The model under review builds one solid part; all positions refer to its coordinate system, in mm. A direction names the side the tool comes from. Round coordinates to 2 decimals unless told otherwise and drop trailing zeros. Write each loop counter-clockwise with the first axis right and the second up, starting at its lowest first coordinate (ties: lowest second). Pieces come first, ordered by that corner, then holes. Notation, with made-up numbers: (27, -39.75) - (35, -39.75) arc R13 ccw to (35, -32.75) - close; hole circle Ø1 at (84, 23.5). An arc over 180 degrees is marked (long way). Use one line per item in the form item = value.
from build123d import *

# Parameters (mm, degrees)
BOSS_EXTRUDE1_DEPTH  = 3
SKETCH1_3_R          = 1.6
CUT_EXTRUDE1_DEPTH   = 219.249429386
MNTPATT_LNDGEAR_D    = 3.4
MNTPATT_REARARM_D    = 3.4
MNTPATT_FOREARM_D    = 3.4
FILLET1_R            = 5
FILLET2_R            = 2
M3_CLEARANCE_HOLE4_D = 3.4


with BuildPart() as part:
    # Sketch1 → Boss-Extrude1 (new body)
    with BuildSketch(Plane.XY):
        Polygon((0, 0), (19, 0), (21.979383981, 2.5), (40.979383981, 2.5), (62.987827091, -27.242703843), (50.343119944, -50.531357328), (50.343119944, -94.031357328), (90.343119944, -163.313389631), (66.562485529, -184.725569035), (51.780413009, -178.602634117), (41.565626765, -198.650280911), (29.565626765, -198.650280911), (29.565626765, -177.650280911), (0, -177.650280911), align=None)
    boss_extrude1 = extrude(amount=BOSS_EXTRUDE1_DEPTH)

    # Sketch1<3> → Cut-Extrude1 (cut, through all)
    with BuildSketch(Plane.XY):
        with Locations((6, -4)):
            Circle(SKETCH1_3_R)
        with Locations((48.043119944, -104.047640471)):
            Circle(SKETCH1_3_R)
        with Locations((53.591147617, -139.888439508)):
            Circle(SKETCH1_3_R)
        with Locations((36.065626765, -194.650280911)):
            Circle(SKETCH1_3_R)
        with Locations((24, -172.650280911)):
            Circle(SKETCH1_3_R)
        with Locations((9, -170.650280911)):
            Circle(SKETCH1_3_R)
        with Locations((15.778522962, -34.052256336)):
            Circle(SKETCH1_3_R)
    cut_extrude1 = extrude(amount=CUT_EXTRUDE1_DEPTH, mode=Mode.SUBTRACT)

    # MntPatt-Lndgear (through all)
    with Locations(Plane.XY.offset(3)):
        with Locations((33.343119944, -56.83261542), (41.343119944, -56.83261542), (33.343119944, -87.83261542), (41.343119944, -87.83261542)):
            mntpatt_lndgear = Hole(MNTPATT_LNDGEAR_D / 2)

    # MntPatt-RearArm (through all)
    with Locations(Plane.XY.offset(3)):
        with Locations((55.826108536, -26.810648111), (50.472703455, -19.575936365)):
            mntpatt_reararm = Hole(MNTPATT_REARARM_D / 2)

    # MntPatt_ForeArm (through all)
    with Locations(Plane.XY.offset(3)):
        with Locations((71.326111319, -173.035401095), (64.63780789, -179.057576552)):
            mntpatt_forearm = Hole(MNTPATT_FOREARM_D / 2)

    # Mirror2: Boss-Extrude1, Cut-Extrude1, MntPatt-Lndgear, MntPatt-RearArm, MntPatt_ForeArm across plane
    add(boss_extrude1.mirror(Plane(origin=(0, 0, 3), x_dir=(0, 0, 1), z_dir=(1, 0, 0))))
    add(cut_extrude1.mirror(Plane(origin=(0, 0, 3), x_dir=(0, 0, 1), z_dir=(1, 0, 0))), mode=Mode.SUBTRACT)
    add(mntpatt_lndgear.mirror(Plane(origin=(0, 0, 3), x_dir=(0, 0, 1), z_dir=(1, 0, 0))), mode=Mode.SUBTRACT)
    add(mntpatt_reararm.mirror(Plane(origin=(0, 0, 3), x_dir=(0, 0, 1), z_dir=(1, 0, 0))), mode=Mode.SUBTRACT)
    add(mntpatt_forearm.mirror(Plane(origin=(0, 0, 3), x_dir=(0, 0, 1), z_dir=(1, 0, 0))), mode=Mode.SUBTRACT)

    # Fillet1
    fillet1_edges = [part.edges().sort_by_distance(p)[0] for p in [
        (-40.979383981, 2.5, 1.5),
        (-62.987827091, -27.242703843, 1.5),
        (-50.343119944, -50.531357328, 1.5),
        (-50.343119944, -94.031357328, 1.5),
        (-90.343119944, -163.313389631, 1.5),
        (-66.562485529, -184.725569035, 1.5),
        (-51.780413009, -178.602634117, 1.5),
        (51.780413009, -178.602634117, 1.5),
        (66.562485529, -184.725569035, 1.5),
        (90.343119944, -163.313389631, 1.5),
        (50.343119944, -94.031357328, 1.5),
        (50.343119944, -50.531357328, 1.5),
        (62.987827091, -27.242703843, 1.5),
        (40.979383981, 2.5, 1.5),
    ]]
    fillet(fillet1_edges, radius=FILLET1_R)

    # Fillet2
    fillet2_edges = [part.edges().sort_by_distance(p)[0] for p in [
        (-41.565626765, -198.650280911, 1.5),
        (-29.565626765, -198.650280911, 1.5),
        (-29.565626765, -177.650280911, 1.5),
        (29.565626765, -177.650280911, 1.5),
        (29.565626765, -198.650280911, 1.5),
        (41.565626765, -198.650280911, 1.5),
    ]]
    fillet(fillet2_edges, radius=FILLET2_R)

    # M3 Clearance Hole4 (through all)
    with Locations(Plane.XY.offset(3)):
        with Locations((-15.25, -73.575140456), (15.25, -73.575140456), (15.25, -104.075140456), (-15.25, -104.075140456)):
            Hole(M3_CLEARANCE_HOLE4_D / 2)


solid = part.part
(1) The part is to be moulded in two halves that separate along Y. For faces 4 (the flat face through (-45.955, -190.036, 1.479)), 5 (the flat face through (69.405, -127.047, 1.479)), 6 (the flat face through (-69.405, -127.047, 1.479)), 7 (the flat face through (51.655, -11.928, 1.479)), say which applies: +Y half, -Y half, draft (parallel to the pull), parting line (faces both ways), or undercut.
Geometry results:
face_4 = -Y half
face_5 = undercut
face_6 = undercut
face_7 = +Y half
(2) Insertion check: P1, Ø1.9, axis at x = -24, y = -172.65, coming from the +Z side; P2, Ø0.9, axis at y = -192, z = 1, coming from the -X side; P3, Ø1, axis at y = -24, z = 0.5, coming from the -X side; P4, Ø1, axis at x = -15, z = 1.5, coming from the +Y side. Each pin has a flat end and moves straight along its axis. Give the tip position at first contact, or say it passes through.
Geometry results:
P1 = through
P2 = -45.18
P3 = -60.96
P4 = 0
(3) Add section A-A on z = 0.45. Count the separate pieces of the cut face and the enclosed holes in it, then the cut area to 3 significant figures.
Geometry results:
separate_pieces = 1
enclosed_holes = 34
area = 22,700 mm2
(4) Machinability: for faces 1 (the flat face through (-56.282, -39.593, 1.479)), 2 (the flat face through (-1, -97, 3)), 3 (the flat face through (56.282, -39.593, 1.479)), which of the approach directions +Z, -Z, +X, -X, +Y, -Y give a long, thin tool a straight path to every point of the face, cutting with its end or side? Answer none if there is none.
Geometry results:
face_1 = +Z, -Z, -X
face_2 = +Z, +X, -X, +Y, -Y
face_3 = +Z, -Z, +X
(5) Add section B-B on y = -151.5. Write out the cut boundary in (x, z), then the cut area to 3 significant figures.
Geometry results:
outline = (-83.52, 0) - (83.52, 0) - (83.52, 3) - (-83.52, 3) - close
area = 501 mm2
(6) To check wall thickness, follow L1, parallel to X at y = -174.5, z = 0.95; L2, parallel to X at y = -173.5, z = 1.1; L3, parallel to Y at x = -53, z = 2.6. State the ranges of each line that lie inside material, in increasing order.
Geometry results:
L1 = -77.92 to -72.19, -70.46 to 70.46, 72.19 to 77.92
L2 = -79.03 to -72.96, -69.69 to -25.36, -22.64 to 22.64, 25.36 to 69.69, 72.96 to 79.03
L3 = -180.12 to -141.38, -138.4 to -98.63, -45.64 to -13.74
